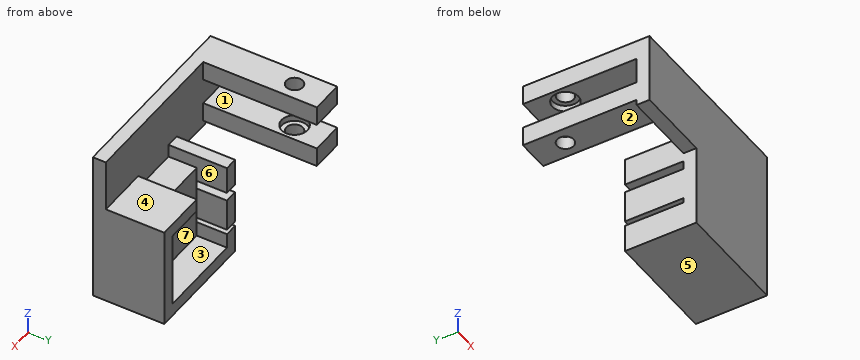
from build123d import *

# Parameters (mm, degrees)
SKETCH1_W           = 60
SKETCH1_H           = 70
BOSS_EXTRUDE1_DEPTH = 4
SKETCH4_W           = 27
SKETCH4_H           = 23.1
BOSS_EXTRUDE3_DEPTH = 8.7
SKETCH3_W           = 10
SKETCH3_H           = 35
SKETCH3_R           = 1.5
BOSS_EXTRUDE2_DEPTH = 6
SKETCH5_W           = 4
SKETCH5_H           = 9.95
SKETCH5_H_2         = 8.45
BOSS_EXTRUDE4_DEPTH = 18
SKETCH6_R           = 2.55
CUT_EXTRUDE1_DEPTH  = 6
SKETCH7_R           = 4
CUT_EXTRUDE2_DEPTH  = 1.9
CUT_EXTRUDE3_REACH  = 6


with BuildPart() as part:
    # Sketch1 → Boss-Extrude1 (new body)
    with BuildSketch(Plane(origin=(0, 0, 0), x_dir=(1, 0, 0), z_dir=(0, 1, 0))):
        with Locations((2.950819672, -17.049180328)):
            Rectangle(SKETCH1_W, SKETCH1_H)
    extrude(amount=BOSS_EXTRUDE1_DEPTH)

    # Sketch4 → Boss-Extrude3 (add)
    with BuildSketch(Plane(origin=(0, 4, 0), x_dir=(1, 0, 0), z_dir=(0, 1, 0))):
        with Locations((15.450819672, -20.499180328)):
            Rectangle(SKETCH4_W, SKETCH4_H)
    extrude(amount=BOSS_EXTRUDE3_DEPTH)

    # Sketch3 → Boss-Extrude2 (add)
    with BuildSketch(Plane.XY.offset(52.049180328)):
        with Locations((-20.249180328, 21.5)):
            Rectangle(SKETCH3_W, SKETCH3_H)
        with Locations((-20.249180328, 29)):
            Circle(SKETCH3_R, mode=Mode.SUBTRACT)
    boss_extrude2 = extrude(amount=-BOSS_EXTRUDE2_DEPTH)

    # Sketch5 → Boss-Extrude4 (add)
    with BuildSketch(Plane(origin=(0, 4, 0), x_dir=(1, 0, 0), z_dir=(0, 1, 0))):
        Polygon((1.950819672, -13.549180328), (1.950819672, -8.949180328), (28.950819672, -8.949180328), (28.950819672, -32.049180328), (16.950819672, -32.049180328), (16.950819672, -36.049180328), (32.950819672, -36.049180328), (32.950819672, -4.949180328), (-2.049180328, -4.949180328), (-2.049180328, -13.549180328), align=None)
        with Locations((-0.049180328, -20.024180328)):
            Rectangle(SKETCH5_W, SKETCH5_H)
        with Locations((-0.049180328, -31.824180328)):
            Rectangle(SKETCH5_W, SKETCH5_H_2)
    extrude(amount=BOSS_EXTRUDE4_DEPTH)

    # Sketch6 → Cut-Extrude1 (cut)
    with BuildSketch(Plane(origin=(0, 0, 46.049180328), x_dir=(-1, 0, 0), z_dir=(0, 0, -1))):
        with Locations((20.249180328, 29)):
            Circle(SKETCH6_R)
    cut_extrude1 = extrude(amount=-CUT_EXTRUDE1_DEPTH, mode=Mode.SUBTRACT)

    # Sketch7 → Cut-Extrude2 (cut)
    with BuildSketch(Plane(origin=(0, 0, 46.049180328), x_dir=(-1, 0, 0), z_dir=(0, 0, -1))):
        with Locations((20.249180328, 29)):
            Circle(SKETCH7_R)
    cut_extrude2 = extrude(amount=-CUT_EXTRUDE2_DEPTH, mode=Mode.SUBTRACT)

    # Mirror1: Boss-Extrude2, Cut-Extrude1, Cut-Extrude2 across plane
    add(boss_extrude2.mirror(Plane(origin=(0, 0, 42.049180328), x_dir=(1, 0, 0), z_dir=(0, 0, -1))))
    add(cut_extrude1.mirror(Plane(origin=(0, 0, 42.049180328), x_dir=(1, 0, 0), z_dir=(0, 0, -1))), mode=Mode.SUBTRACT)
    add(cut_extrude2.mirror(Plane(origin=(0, 0, 42.049180328), x_dir=(1, 0, 0), z_dir=(0, 0, -1))), mode=Mode.SUBTRACT)

    # Sketch9 → Cut-Extrude3 (cut, up to next)
    with BuildSketch(Plane(origin=(0, 4, 0), x_dir=(1, 0, 0), z_dir=(0, 1, 0)), mode=Mode.PRIVATE) as cut_extrude3_sk1:
        Polygon((-2.049180328, -13.549180328), (-2.049180328, -4.949180328), (-27.049180328, -4.949180328), (-27.049180328, -30.311897608), (-25.249180328, -30.311897608), (-2.049180328, -30.311897608), (-2.049180328, -27.599180328), (-2.049180328, -24.999180328), (-2.049180328, -15.049180328), align=None)
    cut_extrude3_tool1 = extrude(cut_extrude3_sk1.sketch, amount=-CUT_EXTRUDE3_REACH, mode=Mode.PRIVATE) & part.part
    add(cut_extrude3_tool1.solids().sort_by_distance((-14.54918, 4, 17.630539))[0], mode=Mode.SUBTRACT)
    # Sketch9 → Cut-Extrude3 (cut, up to next)
    with BuildSketch(Plane(origin=(0, 4, 0), x_dir=(1, 0, 0), z_dir=(0, 1, 0)), mode=Mode.PRIVATE) as cut_extrude3_sk2:
        Polygon((-2.049180328, -4.949180328), (32.950819672, -4.949180328), (32.950819672, 17.950819672), (-27.049180328, 17.950819672), (-27.049180328, -4.949180328), align=None)
    cut_extrude3_tool2 = extrude(cut_extrude3_sk2.sketch, amount=-CUT_EXTRUDE3_REACH, mode=Mode.PRIVATE) & part.part
    add(cut_extrude3_tool2.solids().sort_by_distance((2.95082, 4, -6.50082))[0], mode=Mode.SUBTRACT)
    # Sketch9 → Cut-Extrude3 (cut, up to next)
    with BuildSketch(Plane(origin=(0, 4, 0), x_dir=(1, 0, 0), z_dir=(0, 1, 0)), mode=Mode.PRIVATE) as cut_extrude3_sk3:
        Polygon((-25.249180328, -30.311897608), (-27.049180328, -30.311897608), (-27.049180328, -52.049180328), (-25.249180328, -52.049180328), (-25.249180328, -46.049180328), (-25.249180328, -38.049180328), (-25.249180328, -32.049180328), align=None)
    cut_extrude3_tool3 = extrude(cut_extrude3_sk3.sketch, amount=-CUT_EXTRUDE3_REACH, mode=Mode.PRIVATE) & part.part
    add(cut_extrude3_tool3.solids().sort_by_distance((-26.14918, 4, 41.180539))[0], mode=Mode.SUBTRACT)


solid = part.part
Input: part model. Units: mm. Frame: model coordinates. Face numbers are marked on the shaded views. A direction names the side the tool comes from. Coordinates: 2 decimals unless noted, no trailing zeros. Loops run counter-clockwise (first coordinate to the right, second up) from the corner with the lowest first, then second, coordinate; pieces in that order, holes last.
Q1. Cut plane D-D (x = 20). Output: boundary loops of the cut face in (y, z), then the cut area to 3 significant figures.
Q2. Cut plane A-A (y = 29). Output: boundary loops of the cut face in (x, z).
Q3. Set-up query: the marked faces 1, 2 and 3. Return all of +Z, -Z, +X, -X, +Y, -Y with unobstructed straight access to the full face (end or side cutting, diameter ignored); none if empty.
Q4. Material intervals for line 1 (Z direction, x = 1, y = 7.5); line 2 (Z direction, x = -21, y = 8); line 3 (X direction, y = 14.5, z = 16), sorted ascending.
Q5. Cut plane B-B (y = 18). Output: boundary loops of the cut face in (x, z), then the cut area to 3 significant figures.
Q6. Contact query for flat-ended pins moving along their axis: pin 1 (7 mm diameter, centred on x = -20.25, y = 29, fed in from -Z); pin 2 (4 mm diameter, centred on x = -19.5, y = 29.5, fed in from +Z); pin 3 (4.5 mm diameter, centred on x = -0.5, y = 10, fed in from +Z); pin 4 (4 mm diameter, centred on x = -20.25, y = 29, fed in from +Z). Output: stop coordinate, or through.
Q7. Draft query along Z for the marked faces 4, 5, 6 and 7. Return one class per face: +Z half, -Z half, draft (parallel to the pull), parting line (faces both ways), or undercut.
Q8. Cut plane C-C (z = 34.5). Output: boundary loops of the cut face in (x, y), then the cut area to 3 significant figures.
Working result:
1. outline: (0, 4.95) - (22, 4.95) - (22, 8.95) - (12.7, 8.95) - (12.7, 32.05) - (22, 32.05) - (22, 36.05) - (4, 36.05) - (4, 52.05) - (0, 52.05) - close
1. area: 533 mm2
2. outline: (-25.25, 32.05) - (-22.8, 32.05) - (-22.8, 36.15) - (-24.25, 36.15) - (-24.25, 38.05) - (-25.25, 38.05) - close; (-25.25, 46.05) - (-24.25, 46.05) - (-24.25, 47.95) - (-22.8, 47.95) - (-22.8, 52.05) - (-25.25, 52.05) - close; (-17.7, 32.05) - (-15.25, 32.05) - (-15.25, 38.05) - (-16.25, 38.05) - (-16.25, 36.15) - (-17.7, 36.15) - close; (-17.7, 47.95) - (-16.25, 47.95) - (-16.25, 46.05) - (-15.25, 46.05) - (-15.25, 52.05) - (-17.7, 52.05) - close
3. face 1: +X, -X, +Y
3. face 2: -Z, -X, +Y
3. face 3: +Y
4. line 1: z = 4.95 to 13.55, 15.05 to 25, 27.6 to 36.05
4. line 2: z = 32.05 to 38.05, 46.05 to 52.05
4. line 3: x = -2.05 to 1.95, 28.95 to 32.95
5. outline: (-25.25, 32.05) - (-15.25, 32.05) - (-15.25, 38.05) - (-25.25, 38.05) - close; (-25.25, 46.05) - (-15.25, 46.05) - (-15.25, 52.05) - (-25.25, 52.05) - close; (-2.05, 4.95) - (32.95, 4.95) - (32.95, 36.05) - (16.95, 36.05) - (16.95, 32.05) - (28.95, 32.05) - (28.95, 8.95) - (1.95, 8.95) - (1.95, 13.55) - (-2.05, 13.55) - close; (-2.05, 15.05) - (1.95, 15.05) - (1.95, 25) - (-2.05, 25) - close; (-2.05, 27.6) - (1.95, 27.6) - (1.95, 36.05) - (-2.05, 36.05) - close
5. area: 508 mm2
6. pin 1: stops at z = 32.05
6. pin 2: stops at z = 52.05
6. pin 3: stops at z = 36.05
6. pin 4: passes through
7. face 4: +Z half
7. face 5: -Z half
7. face 6: draft
7. face 7: undercut
8. outline: (-25.25, 0) - (32.95, 0) - (32.95, 22) - (16.95, 22) - (16.95, 4) - (1.95, 4) - (1.95, 22) - (-2.05, 22) - (-2.05, 4) - (-15.25, 4) - (-15.25, 39) - (-25.25, 39) - close; hole circle Ø5.1 at (-20.25, 29)
8. area: 922 mm2
